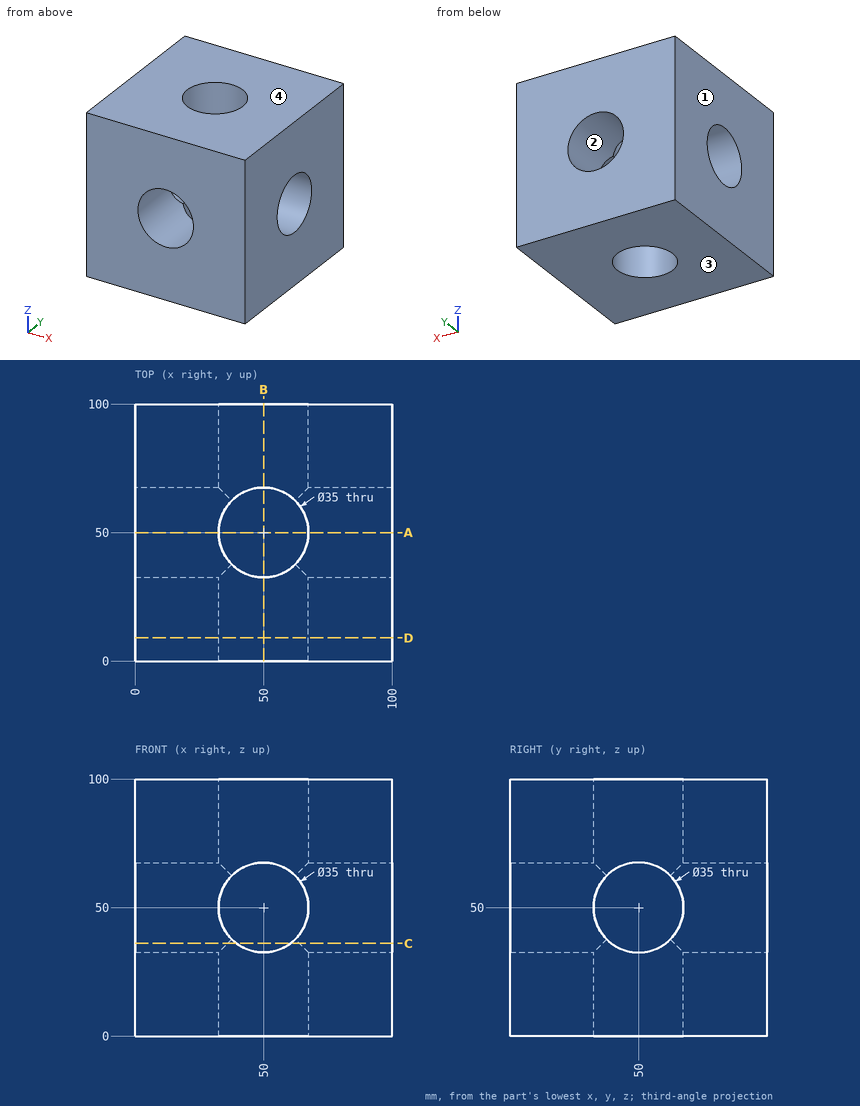
Could you check a few things on this drawing? It's one solid part, dimensions in mm from its lowest x, y, z. Give positions to 0.01 mm unless a question says otherwise; leave off trailing zeros. Order: outer loops, then holes, each group sorted by start corner. A loop starts at its lowest first (then second) coordinate and runs counter-clockwise, first axis right, second up. Notation, with made-up numbers: (36, 76.25) - (46, 76.25) arc R20 cw to (46, 87.25) - close; hole circle Ø6 at (-7.75, 72). An arc over 180 degrees is marked (long way). One line per question, with ' | ' between items. Start each with the question number.
Item 1: I want a section at D-D on y = 9. Write out the boundary of the cut face in (x, z), then the cut area to 3 significant figures.
Item 2: I need wall thicknesses on probe 1 along X at (y, z) = (50, 8). Which ranges of the line are inside material? Lowest first, please. Write a range as [from, to].
Item 3: Thinking about a two-plate mould opening in Z: for the marked faces 1, 2, 3 and 4, which applies, pulls with the +Z half, pulls with the -Z half, needs draft (parallel to the pull), parting line crosses it, or undercut?
Item 4: I want a section at A-A on y = 50. Write out the boundary of the cut face in (x, z).
Item 5: I'm going to push flat-ended pins straight in: pin 1 Ø1 at (x, y) = (87, 61.5) entering from -Z; pin 2 Ø21 at (y, z) = (50, 50) entering from +X. Where does each tip first touch, or does it pass through?
Item 6: I want a section at C-C on z = 36. Write out the boundary of the cut face in (x, y).
Verdict:
1) outline: (0, 0) - (100, 0) - (100, 100) - (0, 100) - close; hole circle Ø35 at (50, 50) | area: 9,040 mm^2
2) probe 1: [0, 32.5], [67.5, 100]
3) face 1: needs draft | face 2: undercut | face 3: pulls with the -Z half | face 4: pulls with the +Z half
4) outline: (0, 0) - (32.5, 0) - (32.5, 32.5) - (0, 32.5) - close; (0, 67.5) - (32.5, 67.5) - (32.5, 100) - (0, 100) - close; (67.5, 0) - (100, 0) - (100, 32.5) - (67.5, 32.5) - close; (67.5, 67.5) - (100, 67.5) - (100, 100) - (67.5, 100) - close
5) pin 1: z = 0 | pin 2: through
6) outline: (0, 0) - (39.5, 0) - (39.5, 36) arc R17.5 cw to (36, 39.5) - (0, 39.5) - close; (0, 60.5) - (36, 60.5) arc R17.5 cw to (39.5, 64) - (39.5, 100) - (0, 100) - close; (60.5, 0) - (100, 0) - (100, 39.5) - (64, 39.5) arc R17.5 cw to (60.5, 36) - close; (60.5, 64) arc R17.5 cw to (64, 60.5) - (100, 60.5) - (100, 100) - (60.5, 100) - close
